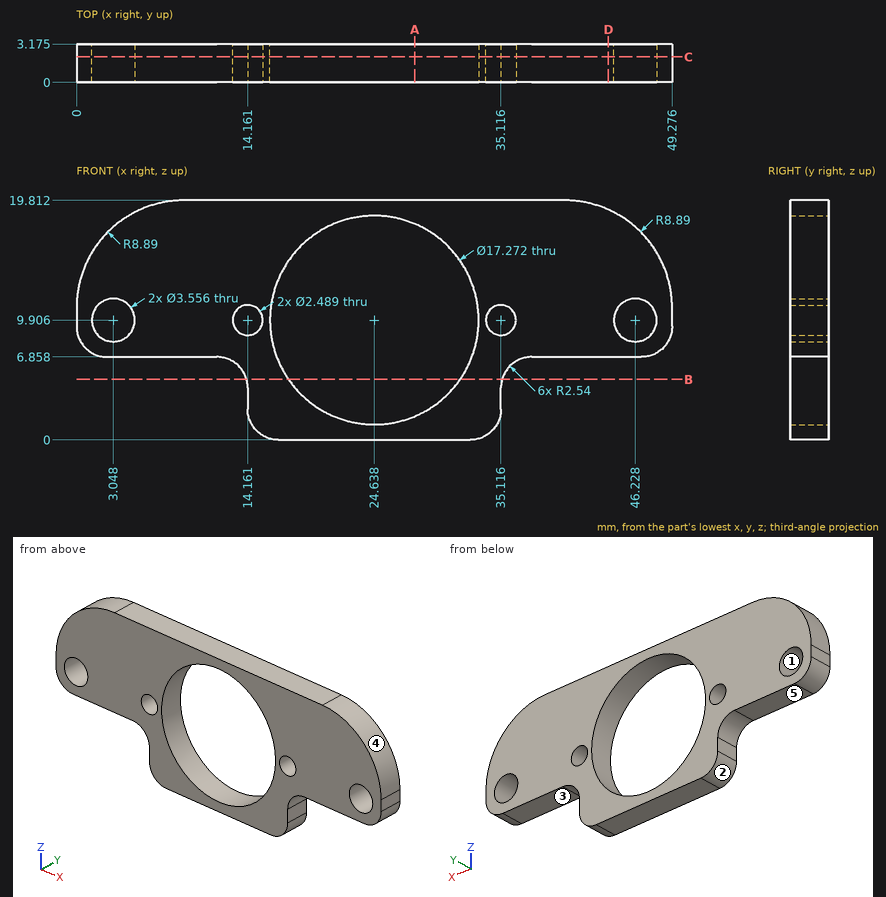
Part print with two shaded views. Sizes in mm from the minimum x, y, z corner. A direction names the side the tool comes from. Coordinates: 2 decimals unless noted, no trailing zeros. Write each loop counter-clockwise with the first axis right and the second up, starting at its lowest first coordinate (ties: lowest second). Pieces come first, ordered by that corner, then holes. Notation, with made-up numbers: M 89.5,40 L 137.5,40 A15 cw 137.5,58 Z; hole C 1.25,86.25 d2. An arc over 180 degrees is marked long. Return JSON: item names as keys, results as strings.
Item 1: Slice it at A-A, the plane x = 28. Write the cut outline in (y, z) (1 decimal).
Findings below:
{"outline": "M 0,0 L 3.2,0 L 3.2,2 L 0,2 Z; M 0,17.9 L 3.2,17.9 L 3.2,19.8 L 0,19.8 Z"}
Item 2: Two-plate mould, pull along X, no slides. Class the marked faces 1, 2 and 3: +X half, -X half, draft (parallel to the pull), parting line (faces both ways), or undercut.
Findings below:
{"face 1": "undercut", "face 2": "-X half", "face 3": "draft"}
Item 3: Slice it at C-C, the plane y = 2.1. Write the cut outline in (x, z) (1 decimal).
Findings below:
{"outline": "M 0,9.4 A2.5 ccw 2.5,6.9 L 11.6,6.9 A2.5 cw 14.2,4.3 L 14.2,2.5 A2.5 ccw 16.7,0 L 32.6,0 A2.5 ccw 35.1,2.5 L 35.1,4.3 A2.5 cw 37.7,6.9 L 46.7,6.9 A2.5 ccw 49.3,9.4 L 49.3,10.9 A8.9 ccw 40.4,19.8 L 8.9,19.8 A8.9 ccw 0,10.9 Z; hole C 3,9.9 d3.6; hole C 14.2,9.9 d2.5; hole C 24.6,9.9 d17.3; hole C 35.1,9.9 d2.5; hole C 46.2,9.9 d3.6"}
Item 4: Slice it at D-D, the plane x = 44. Write the cut outline in (y, z) (1 decimal).
Findings below:
{"outline": "M 0,6.9 L 3.2,6.9 L 3.2,19 L 0,19 Z"}
Item 5: Which spindle directions (+Z, -Z, +X, -X, +Y, -Y) get a long thin tool onto all of the face, cutting with end or side? Do the marked faces 4 and 5. Say none if no direction does.
Findings below:
{"face 4": "+Z, +X, +Y, -Y", "face 5": "-Z, -X, +Y, -Y"}
Item 6: Drop flat-ended pins along their axis: pin 1 Ø4 at (x, z) = (32, 12) entering from +Y (1 decimal); pin 2 Ø1.4 at (y, z) = (2, 3.5) entering from +X (1 decimal); pin 3 Ø1 at (x, y) = (40.5, 2) entering from -Z; pin 4 Ø2 at (x, z) = (14.16, 9.91) entering from +Y. Give the stop position or say it passes through.
Findings below:
{"pin 1": "stops at y = 3.2", "pin 2": "stops at x = 35.1", "pin 3": "stops at z = 6.86", "pin 4": "passes through"}
Item 7: Probe line 1 (X direction, y = 1.4, z = 10) (1 decimal); line 2 (X direction, y = 0.7, z = 11.25) (1 decimal); line 3 (Z direction, x = 14.5, y = 2.35) (1 decimal). List the from-to ranges inside material, lowest first. Write a range as from..to.
Findings below:
{"line 1": "x = 0..1.3, 4.8..12.9, 15.4..16, 33.3..33.9, 36.4..44.5, 48..49.3", "line 2": "x = 0..1.9, 4.2..16.1, 33.2..45.1, 47.4..49.3", "line 3": "z = 1.3..8.7, 11.1..19.8"}
Item 8: Slice it at B-B, the plane z = 5. Write the cut outline in (x, y) (1 decimal), and give its area (3 significant figures).
Findings below:
{"outline": "M 14.1,0 L 17.5,0 L 17.5,3.2 L 14.1,3.2 Z; M 31.7,0 L 35.2,0 L 35.2,3.2 L 31.7,3.2 Z", "area": "22.0 mm2"}
